from build123d import *

# Parameters (mm, degrees)
SKETCH1_R           = 7.5
SKETCH1_R_2         = 1.5
BOSS_EXTRUDE1_DEPTH = 5


with BuildPart() as part:
    # Sketch1 → Boss-Extrude1 (new body)
    with BuildSketch(Plane.XY):
        with BuildLine():
            Line((70, 75), (-70, 75))
            ThreePointArc((-70, 75), (-73.535533906, 73.535533906), (-75, 70))
            Line((-75, 70), (-75, -70))
            ThreePointArc((-75, -70), (-73.535533906, -73.535533906), (-70, -75))
            Line((-70, -75), (70, -75))
            ThreePointArc((70, -75), (73.535533906, -73.535533906), (75, -70))
            Line((75, -70), (75, 70))
            ThreePointArc((75, 70), (73.535533906, 73.535533906), (70, 75))
        make_face()
        with Locations((-60.104076401, 60.104076401)):
            Circle(SKETCH1_R, mode=Mode.SUBTRACT)
        with Locations((60.104076401, 60.104076401)):
            Circle(SKETCH1_R, mode=Mode.SUBTRACT)
        with Locations((60.104076401, -60.104076401)):
            Circle(SKETCH1_R, mode=Mode.SUBTRACT)
        with Locations((-60.104076401, -60.104076401)):
            Circle(SKETCH1_R, mode=Mode.SUBTRACT)
        Circle(SKETCH1_R, mode=Mode.SUBTRACT)
        with Locations((-7.5, 70)):
            Circle(SKETCH1_R_2, mode=Mode.SUBTRACT)
        with Locations((7.5, 70)):
            Circle(SKETCH1_R_2, mode=Mode.SUBTRACT)
        with Locations((70, 7.5)):
            Circle(SKETCH1_R_2, mode=Mode.SUBTRACT)
        with Locations((70, -7.5)):
            Circle(SKETCH1_R_2, mode=Mode.SUBTRACT)
        with Locations((7.5, -70)):
            Circle(SKETCH1_R_2, mode=Mode.SUBTRACT)
        with Locations((-7.5, -70)):
            Circle(SKETCH1_R_2, mode=Mode.SUBTRACT)
        with Locations((-70, -7.5)):
            Circle(SKETCH1_R_2, mode=Mode.SUBTRACT)
        with Locations((-70, 7.5)):
            Circle(SKETCH1_R_2, mode=Mode.SUBTRACT)
        with Locations((40.658639918, 47.72970773)):
            Circle(SKETCH1_R_2, mode=Mode.SUBTRACT)
        with Locations((47.72970773, 40.658639918)):
            Circle(SKETCH1_R_2, mode=Mode.SUBTRACT)
        with Locations((44.194173824, 54.800775542)):
            Circle(SKETCH1_R_2, mode=Mode.SUBTRACT)
        with Locations((54.800775542, 44.194173824)):
            Circle(SKETCH1_R_2, mode=Mode.SUBTRACT)
        with Locations((61.871843354, 47.72970773)):
            Circle(SKETCH1_R_2, mode=Mode.SUBTRACT)
        with Locations((47.72970773, 61.871843354)):
            Circle(SKETCH1_R_2, mode=Mode.SUBTRACT)
        with Locations((51.265241636, 68.942911166)):
            Circle(SKETCH1_R_2, mode=Mode.SUBTRACT)
        with Locations((68.942911166, 51.265241636)):
            Circle(SKETCH1_R_2, mode=Mode.SUBTRACT)
        with Locations((47.72970773, -40.658639918)):
            Circle(SKETCH1_R_2, mode=Mode.SUBTRACT)
        with Locations((54.800775542, -44.194173824)):
            Circle(SKETCH1_R_2, mode=Mode.SUBTRACT)
        with Locations((61.871843354, -47.72970773)):
            Circle(SKETCH1_R_2, mode=Mode.SUBTRACT)
        with Locations((68.942911166, -51.265241636)):
            Circle(SKETCH1_R_2, mode=Mode.SUBTRACT)
        with Locations((51.265241636, -68.942911166)):
            Circle(SKETCH1_R_2, mode=Mode.SUBTRACT)
        with Locations((47.72970773, -61.871843354)):
            Circle(SKETCH1_R_2, mode=Mode.SUBTRACT)
        with Locations((44.194173824, -54.800775542)):
            Circle(SKETCH1_R_2, mode=Mode.SUBTRACT)
        with Locations((40.658639918, -47.72970773)):
            Circle(SKETCH1_R_2, mode=Mode.SUBTRACT)
        with Locations((-40.658639918, -47.72970773)):
            Circle(SKETCH1_R_2, mode=Mode.SUBTRACT)
        with Locations((-44.194173824, -54.800775542)):
            Circle(SKETCH1_R_2, mode=Mode.SUBTRACT)
        with Locations((-47.72970773, -61.871843354)):
            Circle(SKETCH1_R_2, mode=Mode.SUBTRACT)
        with Locations((-51.265241636, -68.942911166)):
            Circle(SKETCH1_R_2, mode=Mode.SUBTRACT)
        with Locations((-68.942911166, -51.265241636)):
            Circle(SKETCH1_R_2, mode=Mode.SUBTRACT)
        with Locations((-61.871843354, -47.72970773)):
            Circle(SKETCH1_R_2, mode=Mode.SUBTRACT)
        with Locations((-54.800775542, -44.194173824)):
            Circle(SKETCH1_R_2, mode=Mode.SUBTRACT)
        with Locations((-47.72970773, -40.658639918)):
            Circle(SKETCH1_R_2, mode=Mode.SUBTRACT)
        with Locations((-47.72970773, 40.658639918)):
            Circle(SKETCH1_R_2, mode=Mode.SUBTRACT)
        with Locations((-54.800775542, 44.194173824)):
            Circle(SKETCH1_R_2, mode=Mode.SUBTRACT)
        with Locations((-61.871843354, 47.72970773)):
            Circle(SKETCH1_R_2, mode=Mode.SUBTRACT)
        with Locations((-68.942911166, 51.265241636)):
            Circle(SKETCH1_R_2, mode=Mode.SUBTRACT)
        with Locations((-51.265241636, 68.942911166)):
            Circle(SKETCH1_R_2, mode=Mode.SUBTRACT)
        with Locations((-47.72970773, 61.871843354)):
            Circle(SKETCH1_R_2, mode=Mode.SUBTRACT)
        with Locations((-44.194173824, 54.800775542)):
            Circle(SKETCH1_R_2, mode=Mode.SUBTRACT)
        with Locations((-40.658639918, 47.72970773)):
            Circle(SKETCH1_R_2, mode=Mode.SUBTRACT)
        with Locations((68.589357775, 68.589357775)):
            Circle(SKETCH1_R_2, mode=Mode.SUBTRACT)
        with Locations((68.589357775, -68.589357775)):
            Circle(SKETCH1_R_2, mode=Mode.SUBTRACT)
        with Locations((-68.589357775, -68.589357775)):
            Circle(SKETCH1_R_2, mode=Mode.SUBTRACT)
        with Locations((-68.589357775, 68.589357775)):
            Circle(SKETCH1_R_2, mode=Mode.SUBTRACT)
        with BuildLine():
            Line((14.142135624, 7.071067812), (36.642135624, 29.571067812))
            ThreePointArc((36.642135624, 29.571067812), (39.886369112, 31.738795325), (43.713203436, 32.5))
            Line((43.713203436, 32.5), (54.713203436, 32.5))
            ThreePointArc((54.713203436, 32.5), (61.784271247, 29.571067812), (64.713203436, 22.5))
            Line((64.713203436, 22.5), (64.713203436, -22.5))
            ThreePointArc((64.713203436, -22.5), (61.784271247, -29.571067812), (54.713203436, -32.5))
            Line((54.713203436, -32.5), (43.713203436, -32.5))
            ThreePointArc((43.713203436, -32.5), (39.886369112, -31.738795325), (36.642135624, -29.571067812))
            Line((36.642135624, -29.571067812), (14.142135624, -7.071067812))
            ThreePointArc((14.142135624, -7.071067812), (11.213203436, 0), (14.142135624, 7.071067812))
        make_face(mode=Mode.SUBTRACT)
        with BuildLine():
            Line((-22.5, 64.713203436), (22.5, 64.713203436))
            ThreePointArc((22.5, 64.713203436), (29.571067812, 61.784271247), (32.5, 54.713203436))
            Line((32.5, 54.713203436), (32.5, 43.713203436))
            ThreePointArc((32.5, 43.713203436), (31.738795325, 39.886369112), (29.571067812, 36.642135624))
            Line((29.571067812, 36.642135624), (7.071067812, 14.142135624))
            ThreePointArc((7.071067812, 14.142135624), (0, 11.213203436), (-7.071067812, 14.142135624))
            Line((-7.071067812, 14.142135624), (-29.571067812, 36.642135624))
            ThreePointArc((-29.571067812, 36.642135624), (-31.738795325, 39.886369112), (-32.5, 43.713203436))
            Line((-32.5, 43.713203436), (-32.5, 54.713203436))
            ThreePointArc((-32.5, 54.713203436), (-29.571067812, 61.784271247), (-22.5, 64.713203436))
        make_face(mode=Mode.SUBTRACT)
        with BuildLine():
            Line((7.071067812, -14.142135624), (29.571067812, -36.642135624))
            ThreePointArc((29.571067812, -36.642135624), (31.738795325, -39.886369112), (32.5, -43.713203436))
            Line((32.5, -43.713203436), (32.5, -54.713203436))
            ThreePointArc((32.5, -54.713203436), (29.571067812, -61.784271247), (22.5, -64.713203436))
            Line((22.5, -64.713203436), (-22.5, -64.713203436))
            ThreePointArc((-22.5, -64.713203436), (-29.571067812, -61.784271247), (-32.5, -54.713203436))
            Line((-32.5, -54.713203436), (-32.5, -43.713203436))
            ThreePointArc((-32.5, -43.713203436), (-31.738795325, -39.886369112), (-29.571067812, -36.642135624))
            Line((-29.571067812, -36.642135624), (-7.071067812, -14.142135624))
            ThreePointArc((-7.071067812, -14.142135624), (0, -11.213203436), (7.071067812, -14.142135624))
        make_face(mode=Mode.SUBTRACT)
        with BuildLine():
            Line((-14.142135624, -7.071067812), (-36.642135624, -29.571067812))
            ThreePointArc((-36.642135624, -29.571067812), (-39.886369112, -31.738795325), (-43.713203436, -32.5))
            Line((-43.713203436, -32.5), (-54.713203436, -32.5))
            ThreePointArc((-54.713203436, -32.5), (-61.784271247, -29.571067812), (-64.713203436, -22.5))
            Line((-64.713203436, -22.5), (-64.713203436, 22.5))
            ThreePointArc((-64.713203436, 22.5), (-61.784271247, 29.571067812), (-54.713203436, 32.5))
            Line((-54.713203436, 32.5), (-43.713203436, 32.5))
            ThreePointArc((-43.713203436, 32.5), (-39.886369112, 31.738795325), (-36.642135624, 29.571067812))
            Line((-36.642135624, 29.571067812), (-14.142135624, 7.071067812))
            ThreePointArc((-14.142135624, 7.071067812), (-11.213203436, 0), (-14.142135624, -7.071067812))
        make_face(mode=Mode.SUBTRACT)
    extrude(amount=BOSS_EXTRUDE1_DEPTH)


solid = part.part
The listing builds one solid part. Answer for the finished solid, in the listing's coordinates (mm). A direction names the side the tool comes from. Give positions to 0.01 mm unless a question says otherwise; leave off trailing zeros. Write each loop counter-clockwise with the first axis right and the second up, starting at its lowest first coordinate (ties: lowest second). Pieces come first, ordered by that corner, then holes. Notation, with made-up numbers: (3.5, 10.5) -> (33.5, 10.5) arc R22 ccw to (33.5, 36.5) -> close; hole circle Ø5 at (78, 46). An arc over 180 degrees is marked (long way). Use a Markdown table: item, result.
(1) Section C-C, the plane z = 3.2 is taken. Give the number of separate pieces and of enclosed holes in the cut face, then the cut area to 3 significant figures.
Return value:
| item | result |
|---|---|
| separate pieces | 1 |
| enclosed holes | 53 |
| area | 10,800 mm2 |
(2) Section A-A, the plane y = 0 is taken. Determine the outline of the cut face in (x, z).
Return value:
| item | result |
|---|---|
| outline | (-75, 0) -> (-64.71, 0) -> (-64.71, 5) -> (-75, 5) -> close; (-11.21, 0) -> (-7.5, 0) -> (-7.5, 5) -> (-11.21, 5) -> close; (7.5, 0) -> (11.21, 0) -> (11.21, 5) -> (7.5, 5) -> close; (64.71, 0) -> (75, 0) -> (75, 5) -> (64.71, 5) -> close |
(3) Determine the mould class of faces 1 (the cylindrical face through (31.76, 39.94, 2.46)), 2 (the flat face through (1, 75, 2)), 3 (the flat face through (-32.5, -49, 2)), 4 (the cylindrical face through (74, 73, 2)) for opening direction X: released by +X, released by -X, zero draft, split by the parting line, or undercut.
Return value:
| item | result |
|---|---|
| face 1 | undercut |
| face 2 | zero draft |
| face 3 | undercut |
| face 4 | released by +X |
(4) Find the intervals of material crossed by probe 1 along Y at (x, z) = (0, 3.15); probe 2 along X at (y, z) = (45, 0.5); probe 3 along X at (y, z) = (-19, 0.45), in increasing order. Write a range as from..to.
Return value:
| item | result |
|---|---|
| probe 1 | -75..-64.71, -11.21..-7.5, 7.5..11.21, 64.71..75 |
| probe 2 | -75..-56.07, -53.54..-32.5, 32.5..53.54, 56.07..75 |
| probe 3 | -75..-64.71, -26.07..-11.93, 11.93..26.07, 64.71..75 |
(5) For faces 5 (the flat face through (-75, 1, 2)), 6 (the cylindrical face through (0.11, 11.214, 2.465)), determine the directions among +Z, -Z, +X, -X, +Y, -Y from which every point of the face is accessible in a straight line to the end or side of a thin tool.
Return value:
| item | result |
|---|---|
| face 5 | +Z, -Z, -X, +Y, -Y |
| face 6 | +Z, -Z |
(6) A flat-ended cylindrical pin translates along its axis: P1, Ø2.5, axis at x = 44.19, y = 54.8, coming from the -Z side. Find the tip coordinate at first contact, or state that the pin passes through.
Return value:
| item | result |
|---|---|
| P1 | through |
